Design review of the part built by this model. Coordinates are the model's own, in mm. A direction names the side the tool comes from. Give positions to 0.01 mm unless a question says otherwise; leave off trailing zeros. Loops run counter-clockwise (first coordinate to the right, second up) from the corner with the lowest first, then second, coordinate; pieces in that order, holes last. Notation, with made-up numbers: (50, 58) -> (96, 58) arc R27 cw to (96, 95) -> close; hole circle Ø9 at (70.5, 26.25). An arc over 180 degrees is marked (long way). Use CSV: the item, a comma, the result in double quotes. Start each with the question number.
Item 1: Wall thickness on line 1 along Y through (x, z) = (-13, -13); line 2 along Y through (x, z) = (-12.2, -5.5); line 3 along Y through (x, z) = (-38.5, 6.5): over which ranges is each line inside the solid? List them lowest first. Write a range as from..to.
Item 2: We need section A-A (x = 6). State the section outline as (y, z) points, plus the area to 3 significant figures.
Item 3: The part is to be moulded in two halves that separate along Z. For faces 5 (the face through (0.028, 13.36, -12.675)), 6 (the face through (-33, 48.5, 5)), 7 (the face through (-66, 44.9, 3)), say which applies: +Z half, -Z half, draft (parallel to the pull), parting line (faces both ways), or undercut.
Item 4: For faces 1 (the face through (-45.5, 46.5, 5)), 2 (the face through (-5.324, 1.726, -7.146)), 3 (the face through (-10, 9, 4)), 4 (the face through (-27, 45, 5)), list the 3-axis set-ups (+Z, -Z, +X, -X, +Y, -Y) from which the entire face can be reached by the end or side of a thin tool; tool diameter is ignored.
Item 5: We need section D-D (x = -6). State the section outline as (y, z) points, plus the area to 3 significant figures.
Item 6: We need section B-B (z = -13). State the section outline as (x, y) points, plus the area to 3 significant figures.
Item 7: Clearance check with flat-ended pins moving along their axes: pin 1 (8 mm diameter, centred on x = -3, z = -20, fed in from -Y); pin 2 (1.5 mm diameter, centred on y = 37.5, z = -12, fed in from -X) (3 decimals); pin 3 (9 mm diameter, centred on x = -5, z = -18.5, fed in from +Y); pin 4 (1.5 mm diameter, centred on y = 35.5, z = -14, fed in from +X). State where each tip first meets the part, or that it passes through.
Item 8: We need section C-C (x = -31.5). State the section outline as (y, z) points, plus the area to 3 significant figures.
from build123d import *

# Parameters (mm, degrees)
BOSS_EXTRUDE1_DEPTH = 10
SKETCH6_W           = 20
SKETCH6_H           = 25
BOSS_EXTRUDE3_DEPTH = 3.5
SKETCH8_R           = 2.25
CUT_EXTRUDE2_DEPTH  = 47.313496953
SKETCH9_W           = 24
SKETCH9_H           = 13
BOSS_EXTRUDE4_DEPTH = 6
SKETCH10_R          = 1.1
CUT_EXTRUDE3_DEPTH  = 2
SKETCH11_R          = 1
CUT_EXTRUDE4_DEPTH  = 51.189042629
SKETCH12_W          = 6
SKETCH12_H          = 2
BOSS_EXTRUDE5_DEPTH = 10
SKETCH14_W          = 4
SKETCH14_H          = 2
CUT_EXTRUDE5_DEPTH  = 2
BOSS_EXTRUDE6_DEPTH = 2
FILLET1_R           = 2
CHAMFER1_SIZE       = 2
CHAMFER2_SIZE       = 10


with BuildPart() as part:
    # Sketch1 → Boss-Extrude1 (new body)
    with BuildSketch(Plane.XY):
        Polygon((-13.7, 36.5), (-13.7, 23.5), (-10, 23.5), (-10, 0), (10, 0), (10, 36.5), align=None)
    extrude(amount=BOSS_EXTRUDE1_DEPTH)

    # Sketch6 → Boss-Extrude3 (add)
    with BuildSketch(Plane.XZ):
        with Locations((0, -12.5)):
            Rectangle(SKETCH6_W, SKETCH6_H)
    extrude(amount=-BOSS_EXTRUDE3_DEPTH)

    # Sketch8 → Cut-Extrude2 (cut, through all)
    with BuildSketch(Plane.XZ):
        with Locations(Location((-6, -5, 0), (0, 0, 270))):
            Circle(SKETCH8_R)
        with Locations(Location((6, -5, 0), (0, 0, 270))):
            Circle(SKETCH8_R)
        with Locations(Location((6, -21, 0), (0, 0, 270))):
            Circle(SKETCH8_R)
        with Locations(Location((-6, -21, 0), (0, 0, 270))):
            Circle(SKETCH8_R)
    extrude(amount=-CUT_EXTRUDE2_DEPTH, mode=Mode.SUBTRACT)

    # Sketch9 → Boss-Extrude4 (add)
    with BuildSketch(Plane.ZY.offset(13.7)):
        with Locations((-12, 30)):
            Rectangle(SKETCH9_W, SKETCH9_H)
    extrude(amount=-BOSS_EXTRUDE4_DEPTH)

    # Sketch10 → Cut-Extrude3 (cut)
    with BuildSketch(Plane.ZY.offset(13.7)):
        with Locations((-13, 34.2)):
            Circle(SKETCH10_R)
        with Locations((-13, 27.8)):
            Circle(SKETCH10_R)
    extrude(amount=-CUT_EXTRUDE3_DEPTH, mode=Mode.SUBTRACT)

    # Sketch11 → Cut-Extrude4 (cut, through all)
    with BuildSketch(Plane.ZY.offset(13.7)):
        with Locations((-20.5, 33.5)):
            Circle(SKETCH11_R)
        with Locations((-5.5, 33.5)):
            Circle(SKETCH11_R)
    extrude(amount=-CUT_EXTRUDE4_DEPTH, mode=Mode.SUBTRACT)

    # Sketch12 → Boss-Extrude5 (add)
    with BuildSketch(Plane.XY.offset(10)):
        Polygon((10, 36.5), (-13.7, 36.5), (-13.7, 33.5), (-44.613248654, 33.5), (-47.5, 38.5), (-47.5, 44.5), (-62.5, 44.5), (-62.5, 42.5), (-66.5, 42.5), (-66.5, 48.5), (10, 48.5), align=None)
        with Locations((-30, 45.5)):
            Rectangle(SKETCH12_W, SKETCH12_H, mode=Mode.SUBTRACT)
        with Locations((-5, 45.5)):
            Rectangle(SKETCH12_W, SKETCH12_H, mode=Mode.SUBTRACT)
    extrude(amount=-BOSS_EXTRUDE5_DEPTH)

    # Sketch14 → Cut-Extrude5 (cut, symmetric)
    with BuildSketch(Plane.XY.offset(5)):
        with Locations((-64.5, 43.5)):
            Rectangle(SKETCH14_W, SKETCH14_H)
        with BuildLine():
            Line((-47.5, 44.5), (-47.5, 42.5))
            ThreePointArc((-47.5, 42.5), (-44.035898385, 44.5), (-44.035898385, 48.5))
            Line((-44.035898385, 48.5), (-47.5, 48.5))
            ThreePointArc((-47.5, 48.5), (-45.5, 46.5), (-47.5, 44.5))
        make_face()
    extrude(amount=CUT_EXTRUDE5_DEPTH, both=True, mode=Mode.SUBTRACT)

    # Sketch15 → Boss-Extrude6 (add, symmetric)
    with BuildSketch(Plane(origin=(0, 0, 0), x_dir=(0, 0, -1), z_dir=(1, 0, 0))):
        Polygon((0, 3.5), (25, 3.5), (0, 23.5), align=None)
    extrude(amount=BOSS_EXTRUDE6_DEPTH, both=True)

    # Fillet1
    fillet1_edges = [part.edges().sort_by_distance(p)[0] for p in [
        (-66.5, 44.5, 5),
        (-66.5, 48.5, 5),
    ]]
    fillet(fillet1_edges, radius=FILLET1_R - 0.0001)  # a hair under: the kernel refuses the full size

    # Chamfer1
    chamfer1_edges = [part.edges().sort_by_distance(p)[0] for p in [
        (-64.5, 42.5, 3),
    ]]
    chamfer(chamfer1_edges, length=CHAMFER1_SIZE - 0.0001)  # a hair under: the kernel refuses the full size

    # Chamfer2
    chamfer2_edges = [part.edges().sort_by_distance(p)[0] for p in [
        (10, 48.5, 5),
    ]]
    chamfer(chamfer2_edges, length=CHAMFER2_SIZE)


solid = part.part
Results found:
1,line 1,"23.5..26.7, 28.9..33.1, 35.3..36.5"
1,line 2,"23.5..32.5, 34.5..36.5"
1,line 3,"33.5..48.5"
2,outline,"(0, -25) -> (3.5, -25) -> (3.5, -23.25) -> (0, -23.25) -> close; (0, -18.75) -> (3.5, -18.75) -> (3.5, -7.25) -> (0, -7.25) -> close; (0, -2.75) -> (3.5, -2.75) -> (3.5, 0) -> (42.5, 0) -> (42.5, 10) -> (0, 10) -> close"
2,area,"481 mm²"
3,face 5,"-Z half"
3,face 6,"draft"
3,face 7,"undercut"
4,face 1,"none"
4,face 2,"-Y"
4,face 3,"+Z, -Z, -X, -Y"
4,face 4,"+Z, -Z"
5,outline,"(0, -25) -> (3.5, -25) -> (3.5, -23.25) -> (0, -23.25) -> close; (0, -18.75) -> (3.5, -18.75) -> (3.5, -7.25) -> (0, -7.25) -> close; (0, -2.75) -> (3.5, -2.75) -> (3.5, 0) -> (44.5, 0) -> (44.5, 10) -> (0, 10) -> close; (46.5, 0) -> (48.5, 0) -> (48.5, 10) -> (46.5, 10) -> close"
5,area,"521 mm²"
6,outline,"(-13.7, 23.5) -> (-7.7, 23.5) -> (-7.7, 36.5) -> (-13.7, 36.5) -> (-13.7, 35.3) -> (-11.7, 35.3) -> (-11.7, 33.1) -> (-13.7, 33.1) -> (-13.7, 28.9) -> (-11.7, 28.9) -> (-11.7, 26.7) -> (-13.7, 26.7) -> close; (-10, 0) -> (10, 0) -> (10, 3.5) -> (2, 3.5) -> (2, 13.1) -> (-2, 13.1) -> (-2, 3.5) -> (-10, 3.5) -> close"
6,area,"178 mm²"
7,pin 1,"y = 0"
7,pin 2,"through"
7,pin 3,"y = 36.5"
7,pin 4,"x = -7.7"
8,outline,"(33.5, 0) -> (44.5, 0) -> (44.5, 10) -> (33.5, 10) -> close; (46.5, 0) -> (48.5, 0) -> (48.5, 10) -> (46.5, 10) -> close"
8,area,"130 mm²"
